Source: CAD feature listing. Evaluate the final solid. Frame: model axes, mm. Coordinates: 2 decimals unless noted, no trailing zeros. Loops run counter-clockwise (first coordinate to the right, second up) from the corner with the lowest first, then second, coordinate; pieces in that order, holes last. Notation, with made-up numbers: M -13,45 L 12,45 A21 cw 12,80 Z; hole C 89,-14 d9. An arc over 180 degrees is marked long. Write each question's results on one line, items separated by ' | '. Start each with the question number.
Autodesk Inventor part; units mm, degrees
ref_plane "YZ Plane" through (0, 0, 0) normal (1, 0, 0) x (0, 1, 0)
ref_plane "XZ Plane" through (0, 0, 0) normal (0, 1, 0) x (-1, 0, 0)
ref_plane "XY Plane" through (0, 0, 0) normal (0, 0, 1) x (1, 0, 0)
sketch "Sketch1" plane through (0, 0, 0) normal (0, 0, 1) x (1, 0, 0)
  line L0 (-30, -18) -> (-30, 12)
  line L1 (-30, 12) -> (120, 12)
  line L2 (120, 12) -> (120, -18)
  line L3 (120, -18) -> (-30, -18)
  point P0 (-30, -3)
  dimension "d13" = 30
  dimension "d55" = 150
extrude "Extrusion1" add sketch "Sketch1" along normal blind 2.8
sketch "Sketch4" plane through (0, 0, 2.8) normal (0, 0, 1) x (1, 0, 0)
  line L0 (-22.4, 6.9) -> (17.9, 6.9)
  line L1 (17.9, -0.5) -> (23.9, -0.5)
  line L2 (17.9, -12.9) -> (-22.4, -12.9)
  line L3 (17.9, -5.5) -> (17.9, -12.9)
  line L4 (17.9, -5.5) -> (17.9, -12.9)
  line L5 (23.9, -5.5) -> (17.9, -5.5)
  line L6 (-22.4, -12.9) -> (-22.4, 6.9)
  line L7 (23.9, -0.5) -> (23.9, -5.5)
  line L8 (17.9, 6.9) -> (17.9, -0.5)
  circle A0 centre (-26.75, -8) radius 2.5
  circle A1 centre (-26.75, 2) radius 2.5
  circle A2 centre (22.25, -8) radius 2.5
  circle A3 centre (22.25, 2) radius 2.5
  circle A4 centre (22.25, -8) radius 1.5
  circle A5 centre (22.25, 2) radius 1.5
  circle A6 centre (-26.75, -8) radius 1.5
  circle A7 centre (-26.75, 2) radius 1.5
  line L9 (120, 12) -> (120, -18)
  line L10 (-30, -18) -> (-30, 12)
  line L11 (120, -18) -> (-30, -18)
  line L12 (120, -3) -> (-30, -3)
  line L13 (112.8, -0.5) -> (115, -0.5)
  line L14 (115, -0.5) -> (115, -5.5)
  line L15 (115, -5.5) -> (112.8, -5.5)
  line L16 (112.8, -5.5) -> (112.8, -0.5)
  line L17 (97.8, -0.5) -> (100, -0.5)
  line L18 (100, -0.5) -> (100, -5.5)
  line L19 (100, -5.5) -> (97.8, -5.5)
  line L20 (97.8, -5.5) -> (97.8, -0.5)
  line L21 (82.8, -0.5) -> (85, -0.5)
  line L22 (85, -0.5) -> (85, -5.5)
  line L23 (85, -5.5) -> (82.8, -5.5)
  line L24 (82.8, -5.5) -> (82.8, -0.5)
  line L25 (67.8, -0.5) -> (70, -0.5)
  line L26 (70, -0.5) -> (70, -5.5)
  line L27 (70, -5.5) -> (67.8, -5.5)
  line L28 (67.8, -5.5) -> (67.8, -0.5)
  line L29 (52.8, -0.5) -> (55, -0.5)
  line L30 (55, -0.5) -> (55, -5.5)
  line L31 (55, -5.5) -> (52.8, -5.5)
  line L32 (52.8, -5.5) -> (52.8, -0.5)
  line L33 (37.8, -0.5) -> (40, -0.5)
  line L34 (40, -0.5) -> (40, -5.5)
  line L35 (40, -5.5) -> (37.8, -5.5)
  line L36 (37.8, -5.5) -> (37.8, -0.5)
  line L37 (112.8, -10.5) -> (115, -10.5)
  line L38 (115, -10.5) -> (115, -15.5)
  line L39 (115, -15.5) -> (112.8, -15.5)
  line L40 (112.8, -15.5) -> (112.8, -10.5)
  line L41 (97.8, -10.5) -> (100, -10.5)
  line L42 (100, -10.5) -> (100, -15.5)
  line L43 (100, -15.5) -> (97.8, -15.5)
  line L44 (97.8, -15.5) -> (97.8, -10.5)
  line L45 (82.8, -10.5) -> (85, -10.5)
  line L46 (85, -10.5) -> (85, -15.5)
  line L47 (85, -15.5) -> (82.8, -15.5)
  line L48 (82.8, -15.5) -> (82.8, -10.5)
  line L49 (67.8, -10.5) -> (70, -10.5)
  line L50 (70, -10.5) -> (70, -15.5)
  line L51 (70, -15.5) -> (67.8, -15.5)
  line L52 (67.8, -15.5) -> (67.8, -10.5)
  line L53 (52.8, -10.5) -> (55, -10.5)
  line L54 (55, -10.5) -> (55, -15.5)
  line L55 (55, -15.5) -> (52.8, -15.5)
  line L56 (52.8, -15.5) -> (52.8, -10.5)
  line L57 (37.8, -10.5) -> (40, -10.5)
  line L58 (40, -10.5) -> (40, -15.5)
  line L59 (40, -15.5) -> (37.8, -15.5)
  line L60 (37.8, -15.5) -> (37.8, -10.5)
  line L61 (112.8, 9.5) -> (112.8, 4.5)
  line L62 (115, 4.5) -> (115, 9.5)
  line L63 (115, 9.5) -> (112.8, 9.5)
  line L64 (112.8, 4.5) -> (115, 4.5)
  line L65 (97.8, 9.5) -> (97.8, 4.5)
  line L66 (100, 4.5) -> (100, 9.5)
  line L67 (100, 9.5) -> (97.8, 9.5)
  line L68 (97.8, 4.5) -> (100, 4.5)
  line L69 (82.8, 9.5) -> (82.8, 4.5)
  line L70 (85, 4.5) -> (85, 9.5)
  line L71 (85, 9.5) -> (82.8, 9.5)
  line L72 (82.8, 4.5) -> (85, 4.5)
  line L73 (67.8, 9.5) -> (67.8, 4.5)
  line L74 (70, 4.5) -> (70, 9.5)
  line L75 (70, 9.5) -> (67.8, 9.5)
  line L76 (67.8, 4.5) -> (70, 4.5)
  line L77 (52.8, 9.5) -> (52.8, 4.5)
  line L78 (55, 4.5) -> (55, 9.5)
  line L79 (55, 9.5) -> (52.8, 9.5)
  line L80 (52.8, 4.5) -> (55, 4.5)
  line L81 (37.8, 9.5) -> (37.8, 4.5)
  line L82 (40, 4.5) -> (40, 9.5)
  line L83 (40, 9.5) -> (37.8, 9.5)
  line L84 (37.8, 4.5) -> (40, 4.5)
  circle A8 centre (106.4, -3) radius 1.5
  circle A9 centre (91.4, -3) radius 1.5
  circle A10 centre (76.4, -3) radius 1.5
  circle A11 centre (61.4, -3) radius 1.5
  circle A12 centre (46.4, -3) radius 1.5
  dimension "d51" = 3
  dimension "d52" = 3
  dimension "d53" = 3
  dimension "d54" = 3
  dimension "d56" = 2.2
  dimension "d57" = 5
  dimension "d58" = 2.5
  dimension "d59" = 5
  dimension "d62" = 15
  dimension "d65" = 10
  dimension "d68" = 3
  dimension "d69" = 6.4
  dimension "d72" = 15
extrude "Extrusion3" cut sketch "Sketch4" against normal blind 10 contours L0 L8 L1 L7 L12 L6 | L12 L7 L5 L3 L2 L6 | L36 L33 L34 L12 | L12 L34 L35 L36 | A12 L12 | L12 A12 | L14 L15 L16 L12 | L12 L16 L13 L14 | L32 L29 L30 L12 | L12 L30 L31 L32 | A8 L12 | L12 A8 | A11 L12 | L12 A11 | L18 L19 L20 L12 | L12 L20 L17 L18 | L28 L25 L26 L12 | L12 L26 L27 L28 | A9 L12 | L12 A9 | A10 L12 | L12 A10 | L22 L23 L24 L12 | L12 L24 L21 L22 | A4 | A5 | A6 | A7 | L37 L38 L39 L40 | L41 L42 L43 L44 | L45 L46 L47 L48 | L49 L50 L51 L52 | L53 L54 L55 L56 | L57 L58 L59 L60 | L63 L62 L64 L61 | L67 L66 L68 L65 | L71 L70 L72 L69 | L75 L74 L76 L73 | L79 L78 L80 L77 | L83 L82 L84 L81
properties part number "Acrylic_UpperArm"
Item 1: Cut plane D-D (x = 0.5). Output: boundary loops of the cut face in (y, z).
Item 2: Mould query, pull axis X, two halves, no side actions, for faces 1 (the flat face through (44, -3, 2.8)), 2 (the flat face through (52.8, 7, 1)), 3 (the flat face through (97.8, 7, 1)). Classes: +X half, -X half, draft (parallel to the pull), parting line (faces both ways), or undercut.
Item 3: Cut plane B-B (x = -26.75). Output: boundary loops of the cut face in (y, z).
Item 4: Cut plane A-A (x = 19.5). Output: boundary loops of the cut face in (y, z).
Item 5: Cut plane C-C (y = -8). Output: boundary loops of the cut face in (x, z).
Item 6: Line query: probe 1 along Y at (x, z) = (54, 0.9); probe 2 along Y at (x, z) = (22.25, 0.7); probe 3 along X at (y, z) = (0, 1.55). Output: solid intervals per line, ascending.
Response values:
1) outline: M -18,0 L -12.9,0 L -12.9,2.8 L -18,2.8 Z; M 6.9,0 L 12,0 L 12,2.8 L 6.9,2.8 Z
2) face 1: draft | face 2: undercut | face 3: undercut
3) outline: M -18,0 L -9.5,0 L -9.5,2.8 L -18,2.8 Z; M -6.5,0 L 0.5,0 L 0.5,2.8 L -6.5,2.8 Z; M 3.5,0 L 12,0 L 12,2.8 L 3.5,2.8 Z
4) outline: M -18,0 L -5.5,0 L -5.5,2.8 L -18,2.8 Z; M -0.5,0 L 12,0 L 12,2.8 L -0.5,2.8 Z
5) outline: M -30,0 L -28.25,0 L -28.25,2.8 L -30,2.8 Z; M -25.25,0 L -22.4,0 L -22.4,2.8 L -25.25,2.8 Z; M 17.9,0 L 20.75,0 L 20.75,2.8 L 17.9,2.8 Z; M 23.75,0 L 120,0 L 120,2.8 L 23.75,2.8 Z
6) probe 1: y = -18 to -15.5, -10.5 to -5.5, -0.5 to 4.5, 9.5 to 12 | probe 2: y = -18 to -9.5, -6.5 to -5.5, -0.5 to 0.5, 3.5 to 12 | probe 3: x = -30 to -22.4, 17.9 to 120
